For this review, take the finished solid that the model builds, in its own axes (mm). A direction names the side the tool comes from. Coordinates: 2 decimals unless noted, no trailing zeros. Write each loop counter-clockwise with the first axis right and the second up, starting at its lowest first coordinate (ties: lowest second). Pieces come first, ordered by that corner, then holes.
```python
from build123d import *

# Parameters (mm, degrees)
F1_DEPTH = 4
F2_R     = 2.25
F3_DEPTH = 25
F6_SIZE  = 1


with BuildPart() as f1:
    # F0 (on Front) → F1 (new body)
    with BuildSketch(Plane.XZ):
        Polygon((2.020726, 3.5), (-2.020726, 3.5), (-4.041452, 0), (-2.020726, -3.5), (2.020726, -3.5), (4.041452, 0), align=None)
    extrude(amount=F1_DEPTH)

    # F2 (on face) → F3 (join)
    with BuildSketch(Plane.XZ.offset(4)):
        Circle(F2_R)
    extrude(amount=F3_DEPTH)

    # F4 (on Top) → F5 (revolve, cut)
    with BuildSketch(Plane.XY):
        with BuildLine():
            Line((-7.239562, -3.979997), (-4.041452, -3.979997))
            Line((-4.041452, -3.979997), (-4.041452, -1.791452))
            ThreePointArc((-4.041452, -1.791452), (-3.516748, -0.524704), (-2.25, 0))
            Line((-2.25, 0), (0, 0))
            Line((0, 0), (0, 3.398254))
            Line((0, 3.398254), (-7.627891, 4.230388))
            Line((-7.627891, 4.230388), (-7.239562, -3.979997))
        make_face()
    revolve(axis=Axis((0, 1.699127, 0), (0, 1, 0)), mode=Mode.SUBTRACT)

    # F6
    f6_edges = [f1.edges().sort_by_distance(p)[0] for p in [
        (-2.25, -29, 0),
    ]]
    chamfer(f6_edges, length=F6_SIZE)


solid = f1.part
```
1) Clearance check with flat-ended pins moving along their axes: P1, Ø4, axis at x = -2.5, y = -15, coming from the +Z side; P2, Ø2, axis at x = 2, y = -17.5, coming from the +Z side; P3, Ø1, axis at x = -3, z = 1, coming from the -Y side. State where each tip first meets the part, or that it passes through.
2) Tool access review of faces 1 (the face through (0, -2, -3.5)), 2 (the face through (2, -4, 2)): name each direction out of +Z, -Z, +X, -X, +Y, -Y from which nothing blocks a thin tool from reaching the whole face with its end or side.
3) Consider section C-C (y = -3.25). Give the boundary of the cut face in (x, z), then the cut area to 3 significant figures.
4) Consider section B-B (y = -15.5). Give the boundary of the cut face in (x, z).
5) For L1, parallel to Z at x = 0, y = -26.25; L2, parallel to Z at x = -1, y = -16.5; L3, parallel to X at y = -26.5, z = -1.75, list the stretches that pass through material, from the lowest coordinate up.
6) Consider section A-A (x = 0). Give the boundary of the cut face in (y, z).
Results:
1. P1: stops at z = 2.19
1. P2: stops at z = 2.02
1. P3: stops at y = -4
2. face 1: -Z, +X, -X, +Y, -Y
2. face 2: -Y
3. outline: (-4.04, 0) - (-2.02, -3.5) - (2.02, -3.5) - (4.04, 0) - (2.02, 3.5) - (-2.02, 3.5) - close
3. area: 42.4 mm2
4. outline: circle Ø4.5 at (0, 0)
5. L1: z = -2.25 to 2.25
5. L2: z = -2.02 to 2.02
5. L3: x = -1.41 to 1.41
6. outline: (-29, -1.25) - (-28, -2.25) - (-4, -2.25) - (-4, -3.5) - (-0.51, -3.5) arc R1.79 ccw to (0, -2.25) - (0, 2.25) arc R1.79 ccw to (-0.51, 3.5) - (-4, 3.5) - (-4, 2.25) - (-28, 2.25) - (-29, 1.25) - close
